CAD build for the part. Positions are in the model's coordinates, mm. A direction names the side the tool comes from. Round coordinates to 2 decimals unless told otherwise and drop trailing zeros. Answer in a Markdown table with one row per item. Add a question column.
```python
from build123d import *

# Parameters (mm, degrees)
SKETCH_1_W          = 47.9
SKETCH_1_H          = 78
EXTRUDE_1_DEPTH     = 3
SKETCH_2_R          = 0.7
CUT_EXTRUDE_1_DEPTH = 46.865046604
SKETCH_2_3_R        = 1
CUT_EXTRUDE_2_DEPTH = 1.5


with BuildPart() as part:
    # 草图1 → 凸台-拉伸1 (new body)
    with BuildSketch(Plane.XY):
        Rectangle(SKETCH_1_W, SKETCH_1_H)
    extrude(amount=EXTRUDE_1_DEPTH)

    # 草图2 → 切除-拉伸1 (cut, through all)
    with BuildSketch(Plane(origin=(0, 0, 0), x_dir=(-1, 0, 0), z_dir=(0, 0, -1))):
        with Locations((-13.95, 37.5)):
            Circle(SKETCH_2_R)
        with Locations((13.95, 37.5)):
            Circle(SKETCH_2_R)
        with Locations((-13.95, -37.5)):
            Circle(SKETCH_2_R)
        with Locations((13.95, -37.5)):
            Circle(SKETCH_2_R)
        with Locations((-22.45, 16)):
            Circle(SKETCH_2_R)
        with Locations((-22.45, -16)):
            Circle(SKETCH_2_R)
        with Locations((22.45, 16)):
            Circle(SKETCH_2_R)
        with Locations((22.45, -16)):
            Circle(SKETCH_2_R)
    extrude(amount=-CUT_EXTRUDE_1_DEPTH, mode=Mode.SUBTRACT)

    # 草图2<3> → 切除-拉伸2 (cut)
    with BuildSketch(Plane(origin=(0, 0, 0), x_dir=(-1, 0, 0), z_dir=(0, 0, -1))):
        with Locations((-13.95, 37.5)):
            Circle(SKETCH_2_3_R)
        with Locations((13.95, 37.5)):
            Circle(SKETCH_2_3_R)
        with Locations((-13.95, -37.5)):
            Circle(SKETCH_2_3_R)
        with Locations((13.95, -37.5)):
            Circle(SKETCH_2_3_R)
        with Locations((-22.45, 16)):
            Circle(SKETCH_2_3_R)
        with Locations((22.45, 16)):
            Circle(SKETCH_2_3_R)
        with Locations((-22.45, -16)):
            Circle(SKETCH_2_3_R)
        with Locations((22.45, -16)):
            Circle(SKETCH_2_3_R)
    extrude(amount=-CUT_EXTRUDE_2_DEPTH, mode=Mode.SUBTRACT)


solid = part.part
```
Item 1: Pin check, flat tip, straight feed: pin 1 (0.6 mm diameter, centred on x = 14, y = 38, fed in from -Z). Stop position of the tip, or through.
Item 2: Drill centre lines: probe 1 along X at (y, z) = (37.5, 2.1); probe 2 along Y at (x, z) = (-13.95, 0.9); probe 3 along Y at (x, z) = (22.45, 0.75). Where is each one in solid material? Low to high.
Item 3: Tool access for faces 1 (the cylindrical face through (-22.233, 15.024, 0.74)), 2 (the cylindrical face through (-22.83, -15.41, 2.24)): list every direction of +Z, -Z, +X, -X, +Y, -Y with a clear straight run to the whole face (end or side of a thin tool).
Item 4: Two-plate mould, pull along Y, no slides. Class faces 3 (the flat face through (0, 39, 1)), 4 (the flat face through (0, -39, 1)), 5 (the flat face through (0, 1, 0)), 6 (the cylindrical face through (22.667, -16.976, 0.74)): +Y half, -Y half, draft (parallel to the pull), parting line (faces both ways), or undercut.
Recorded:
| question | item | result |
|---|---|---|
| 1 | pin 1 | z = 1.5 |
| 2 | probe 1 | -23.95 to -14.65, -13.25 to 13.25, 14.65 to 23.95 |
| 2 | probe 2 | -39 to -38.5, -36.5 to 36.5, 38.5 to 39 |
| 2 | probe 3 | -39 to -17, -15 to 15, 17 to 39 |
| 3 | face 1 | -Z |
| 3 | face 2 | +Z, -Z |
| 4 | face 3 | +Y half |
| 4 | face 4 | -Y half |
| 4 | face 5 | draft |
| 4 | face 6 | undercut |
